Build history of the part. All positions in model axes, mm. Face numbers are marked on the shaded views. A direction names the side the tool comes from. Round coordinates to 2 decimals unless told otherwise and drop trailing zeros. Write each loop counter-clockwise with the first axis right and the second up, starting at its lowest first coordinate (ties: lowest second). Pieces come first, ordered by that corner, then holes. Notation, with made-up numbers: (-18, 22) -> (12, 22) arc R19 ccw to (12, 48) -> close; hole circle Ø6 at (51, 59). An arc over 180 degrees is marked (long way). Answer in a Markdown table with one row per item. Add a question column.
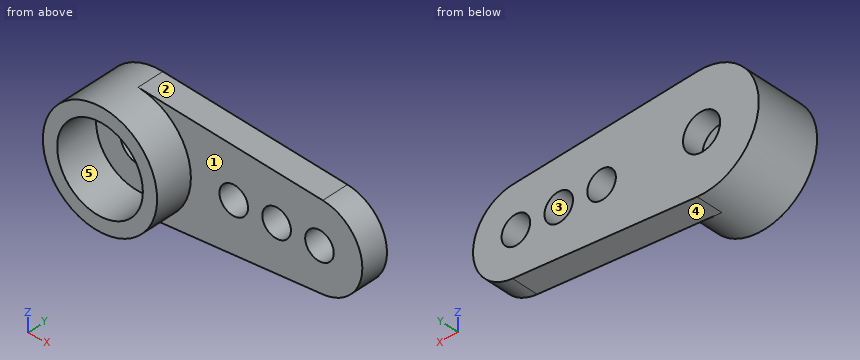
from build123d import *

# Parameters (mm, degrees)
SKETCH_1_R          = 4
SKETCH_1_R_2        = 1.3
EXTRUDE_1_DEPTH     = 4.5
SKETCH_2_R          = 1
EXTRUDE_2_DEPTH     = 1.9
SKETCH_3_R          = 3
CUT_EXTRUDE_1_DEPTH = 3


with BuildPart() as part:
    # 草图1 → 凸台-拉伸1 (new body)
    with BuildSketch(Plane(origin=(0, 0, 0), x_dir=(1, 0, 0), z_dir=(0, 1, 0))):
        Circle(SKETCH_1_R)
        Circle(SKETCH_1_R_2, mode=Mode.SUBTRACT)
    extrude(amount=EXTRUDE_1_DEPTH)

    # 草图2 → 凸台-拉伸2 (add)
    with BuildSketch(Plane(origin=(0, 4.5, 0), x_dir=(1, 0, 0), z_dir=(0, 1, 0))):
        with BuildLine():
            Line((13.230769231, 2.991111092), (0.307692308, 3.988148122))
            ThreePointArc((0.307692308, 3.988148122), (4, 0), (0.307692308, -3.988148122))
            Line((0.307692308, -3.988148122), (13.230769231, -2.991111092))
            ThreePointArc((13.230769231, -2.991111092), (16, 0), (13.230769231, 2.991111092))
        make_face()
        with Locations((10, 0)):
            Circle(SKETCH_2_R, mode=Mode.SUBTRACT)
        with Locations((7, 0)):
            Circle(SKETCH_2_R, mode=Mode.SUBTRACT)
        with Locations((13, 0)):
            Circle(SKETCH_2_R, mode=Mode.SUBTRACT)
    extrude(amount=-EXTRUDE_2_DEPTH)

    # 草图3 → 切除-拉伸1 (cut)
    with BuildSketch(Plane.XZ):
        Circle(SKETCH_3_R)
    extrude(amount=-CUT_EXTRUDE_1_DEPTH, mode=Mode.SUBTRACT)


solid = part.part
(1) Drop flat-ended pins along their axis: P1, Ø4, axis at x = 0, z = 0, coming from the -Y side; P2, Ø1, axis at y = 1, z = -3, coming from the -X side; P3, Ø1, axis at x = 6.5, z = 3, coming from the -Y side; P4, Ø1.8, axis at x = 7, z = 0, coming from the -Y side. Give the stop position or say it passes through.
(2) Saw through at D-D (z = 2). List the corners of the cut face in (x, y).
(3) Which spindle directions (+Z, -Z, +X, -X, +Y, -Y) get a long thin tool onto all of the face, cutting with end or side? Do the marked faces 4 and 5. Say none if no direction does.
(4) Saw through at A-A (x = 0). List the corners of the cut face in (y, z), plus the area to 3 significant figures.
(5) Probe line 1 along Z through (x, y) = (0, 0.8); line 2 along Y through (x, z) = (-1.5, 0.25); line 3 along Z through (x, y) = (13, 3.65). List the from-to ranges inside material, lowest first.
(6) Mould opens along Z. For the marked faces 1, 2 and 3 say: pulls with the +Z half, pulls with the -Z half, needs draft (parallel to the pull), parting line crosses it, or undercut.
(7) Saw through at B-B (z = 0). List the corners of the cut face in (x, y).
(8) Saw through at C-C (y = 2.8). List the corners of the cut face in (x, z).
Answer sheet:
| question | item | result |
|---|---|---|
| 1 | P1 | stops at y = 3 |
| 1 | P2 | stops at x = -3.12 |
| 1 | P3 | stops at y = 2.6 |
| 1 | P4 | passes through |
| 2 | outline | (-3.46, 0) -> (-2.24, 0) -> (-2.24, 3) -> (2.24, 3) -> (2.24, 0) -> (3.46, 0) -> (3.46, 2.6) -> (15.24, 2.6) -> (15.24, 4.5) -> (-3.46, 4.5) -> close |
| 3 | face 4 | -Z, +X, +Y, -Y |
| 3 | face 5 | -Y |
| 4 | outline | (0, -4) -> (4.5, -4) -> (4.5, -1.3) -> (3, -1.3) -> (3, -3) -> (0, -3) -> close; (0, 3) -> (3, 3) -> (3, 1.3) -> (4.5, 1.3) -> (4.5, 4) -> (0, 4) -> close |
| 4 | area | 14.1 mm² |
| 5 | line 1 | z = -4 to -3, 3 to 4 |
| 5 | line 2 | y = 3 to 4.5 |
| 5 | line 3 | z = -3.01 to -1, 1 to 3.01 |
| 6 | face 1 | needs draft |
| 6 | face 2 | pulls with the +Z half |
| 6 | face 3 | undercut |
| 7 | outline | (-4, 0) -> (-3, 0) -> (-3, 3) -> (-1.3, 3) -> (-1.3, 4.5) -> (-4, 4.5) -> close; (1.3, 3) -> (3, 3) -> (3, 0) -> (4, 0) -> (4, 2.6) -> (6, 2.6) -> (6, 4.5) -> (1.3, 4.5) -> close; (8, 2.6) -> (9, 2.6) -> (9, 4.5) -> (8, 4.5) -> close; (11, 2.6) -> (12, 2.6) -> (12, 4.5) -> (11, 4.5) -> close; (14, 2.6) -> (16, 2.6) -> (16, 4.5) -> (14, 4.5) -> close |
| 8 | outline | (0.31, -3.99) -> (13.23, -2.99) arc R3 ccw to (13.23, 2.99) -> (0.31, 3.99) arc R4 ccw (long way) to start; hole circle Ø6 at (0, 0); hole circle Ø2 at (7, 0); hole circle Ø2 at (10, 0); hole circle Ø2 at (13, 0) |
